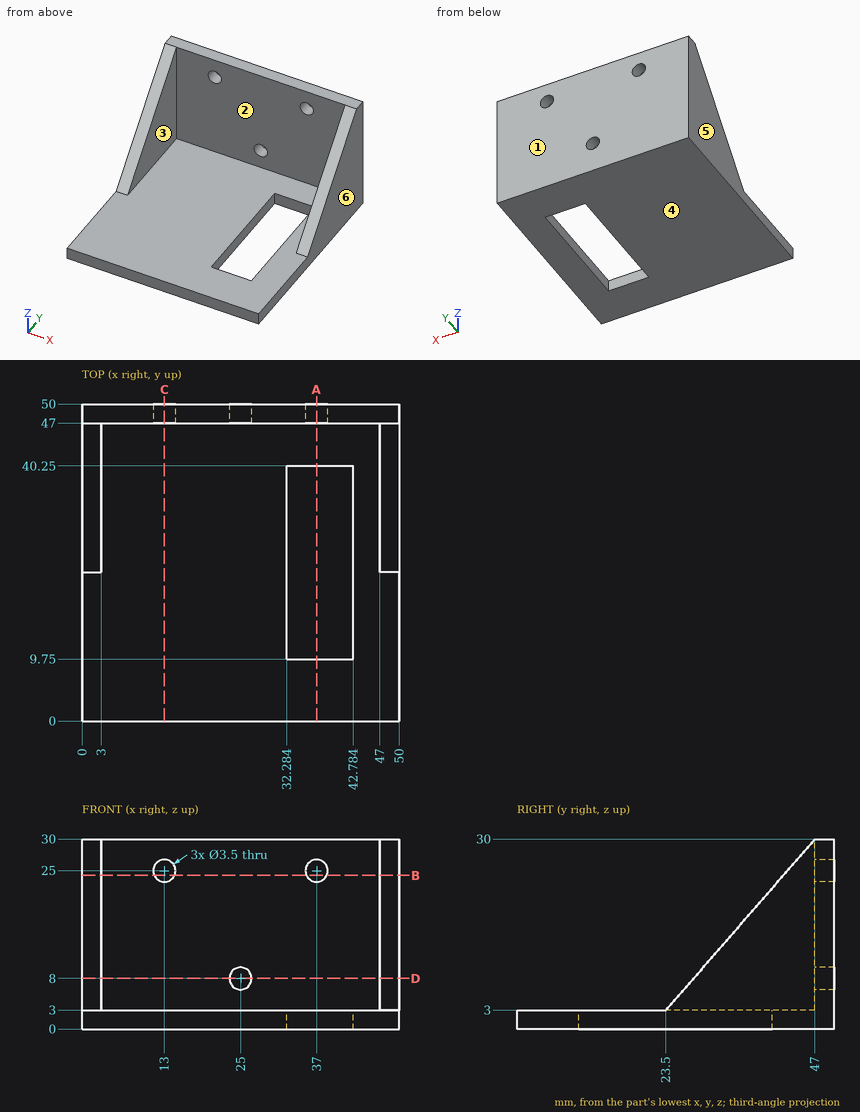
For this review, use the dimensioned drawing (mm, ordinates from the lowest corner) and the shaded views. A direction names the side the tool comes from. Round coordinates to 2 decimals unless told otherwise and drop trailing zeros. Write each loop counter-clockwise with the first axis right and the second up, starting at its lowest first coordinate (ties: lowest second). Pieces come first, ordered by that corner, then holes. Notation, with made-up numbers: (72, 24) - (100, 24) arc R9 ccw to (100, 33) - close; hole circle Ø6 at (20, 52.25). An arc over 180 degrees is marked (long way). One line per item, written item: value. Start each with the question number.
1. Consider section D-D on z = 8. Write out the cut boundary in (x, y), and give its area (3 significant figures).
2. Machinability: for the marked faces 1 and 2, which of the approach directions +Z, -Z, +X, -X, +Y, -Y give a long, thin tool a straight path to every point of the face, cutting with its end or side? Answer none if there is none.
3. The part is to be moulded in two halves that separate along X. For the marked faces 3, 4, 5 and 6, say which applies: released by +X, released by -X, zero draft, split by the parting line, or undercut.
4. Consider section A-A on x = 37. Write out the cut boundary in (y, z).
5. Clearance check with flat-ended pins moving along their axes: P1, Ø3.5, axis at y = 28.5, z = 2, coming from the -X side; P2, Ø1, axis at x = 11.5, z = 11, coming from the -Y side. State where each tip first meets the part, or that it passes through.
6. Consider section C-C on x = 13. Write out the cut boundary in (y, z).
7. To check wall thickness, follow L1, parallel to X at y = 34, z = 11.5; L2, parallel to Z at x = 13, y = 48.15; L3, parallel to Z at x = 43, y = 11. State the ranges of each line that lie inside material, in increasing order. Write a range as from..to.
8. Consider section B-B on z = 24.25. Write out the cut boundary in (x, y) (1 decimal).
Checks:
1. outline: (0, 27.85) - (3, 27.85) - (3, 47) - (23.25, 47) - (23.25, 50) - (0, 50) - close; (26.75, 47) - (47, 47) - (47, 27.85) - (50, 27.85) - (50, 50) - (26.75, 50) - close
1. area: 254 mm^2
2. face 1: +Z, -Z, +X, -X, +Y
2. face 2: +Z, -Y
3. face 3: undercut
3. face 4: zero draft
3. face 5: released by -X
3. face 6: released by +X
4. outline: (0, 0) - (9.75, 0) - (9.75, 3) - (0, 3) - close; (40.25, 0) - (50, 0) - (50, 23.25) - (47, 23.25) - (47, 3) - (40.25, 3) - close; (47, 26.75) - (50, 26.75) - (50, 30) - (47, 30) - close
5. P1: stops at x = 0
5. P2: stops at y = 47
6. outline: (0, 0) - (50, 0) - (50, 23.25) - (47, 23.25) - (47, 3) - (0, 3) - close; (47, 26.75) - (50, 26.75) - (50, 30) - (47, 30) - close
7. L1: x = 0..3, 47..50
7. L2: z = 0..23.25, 26.75..30
7. L3: z = 0..3
8. outline: (0, 42) - (3, 42) - (3, 47) - (11.4, 47) - (11.4, 50) - (0, 50) - close; (14.6, 47) - (35.4, 47) - (35.4, 50) - (14.6, 50) - close; (38.6, 47) - (47, 47) - (47, 42) - (50, 42) - (50, 50) - (38.6, 50) - close
